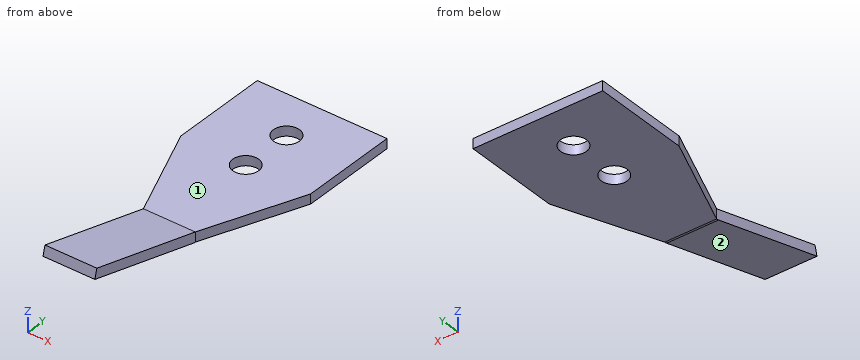
from build123d import *

# Parameters (mm, degrees)
SKETCH1_W           = 200
SKETCH1_H           = 300
SKETCH1_R           = 20
BOSS_EXTRUDE1_DEPTH = 15
CUT_EXTRUDE1_DEPTH  = 15
SKETCH3_W           = 80
SKETCH3_H           = 15
REVOLVE1_ANGLE      = 15
SKETCH4_W           = 80
SKETCH4_H           = 15
BOSS_EXTRUDE3_DEPTH = 200


with BuildPart() as part:
    # Sketch1 → Boss-Extrude1 (new body)
    with BuildSketch(Plane.XY):
        with Locations((-100, 150)):
            Rectangle(SKETCH1_W, SKETCH1_H)
        with Locations((-100, 230)):
            Circle(SKETCH1_R, mode=Mode.SUBTRACT)
        with Locations((-100, 150)):
            Circle(SKETCH1_R, mode=Mode.SUBTRACT)
    extrude(amount=BOSS_EXTRUDE1_DEPTH)

    # Sketch2 → Cut-Extrude1 (cut)
    with BuildSketch(Plane(origin=(0, 0, 0), x_dir=(-1, 0, 0), z_dir=(0, 0, -1))):
        Polygon((0, 0), (60, 0), (0, 150), align=None)
        Polygon((200, 0), (140, 0), (200, 150), align=None)
    extrude(amount=-CUT_EXTRUDE1_DEPTH, mode=Mode.SUBTRACT)

    # Sketch3 → Revolve1 (revolve)
    with BuildSketch(Plane.XZ):
        with Locations((-100, 7.5)):
            Rectangle(SKETCH3_W, SKETCH3_H)
    revolve(axis=Axis((-60, 0, 15), (-1, 0, 0)), revolution_arc=REVOLVE1_ANGLE)

    # Sketch4 → Boss-Extrude3 (add)
    with BuildSketch(Plane(origin=(0, -3.75, 1.004809472), x_dir=(1, 0, 0), z_dir=(0, -0.9659258262890681, 0.25881904510252135))):
        with Locations((-100, 6.988887394)):
            Rectangle(SKETCH4_W, SKETCH4_H)
    extrude(amount=BOSS_EXTRUDE3_DEPTH)


solid = part.part
Verification items for the finished model (mm, model axes). Face numbers are marked on the shaded views. A direction names the side the tool comes from. Give positions to 0.01 mm unless a question says otherwise; leave off trailing zeros. Order: outer loops, then holes, each group sorted by start corner. A loop starts at its lowest first (then second) coordinate and runs counter-clockwise, first axis right, second up. Notation, with made-up numbers: M 84.25,46.25 L 106.25,46.25 A15 ccw 106.25,64.25 Z; hole C -15.75,-21.5 d5. An arc over 180 degrees is marked long. Answer as a JSON object with one key per item and string values. Group by question number.
1) Cross-section at A-A (y = 230). Enter the section's corners in (x, z), then the cut area to 3 significant figures.
2) Cross-section at D-D (x = -67.5). Enter the section's corners in (y, z).
3) Cross-section at B-B (x = -100). Enter the section's corners in (y, z).
4) Access from +Z, -Z, +X, -X, +Y, -Y to the whole of each face (thin tool, end or side, straight path). Record for the marked faces 1 and 2.
5) Scan lines: line 1 along Z through (x, y) = (-13.5, 225); line 2 along X through (y, z) = (247, 5); line 3 along Z through (x, y) = (-108, -82.5). Record each from-to range of solid material in increasing order. Write a range as [from, to].
6) Depth check by flat-ended pin: pin 1 Ø20 at (y, z) = (-54, 27.5) entering from +X; pin 2 Ø8 at (x, y) = (-69.5, 69) entering from +Z. Enter the tip coordinate at first touch or a pass-through.
7) Cross-section at C-C (z = 10). Enter the section's corners in (x, y), then the cut area to 3 significant figures.
Result sheet:
{
 "1": {"outline": "M -200,0 L -120,0 L -120,15 L -200,15 Z; M -80,0 L 0,0 L 0,15 L -80,15 Z", "area": "2,400 mm2"},
 "2": {"outline": "M -197.07,52.27 L -3.88,0.51 A15 ccw 0,0 L 300,0 L 300,15 L 0,15 L -193.19,66.76 Z"},
 "3": {"outline": "M -197.07,52.27 L -3.88,0.51 A15 ccw 0,0 L 130,0 L 130,15 L 0,15 L -193.19,66.76 Z; M 170,0 L 210,0 L 210,15 L 170,15 Z; M 250,0 L 300,0 L 300,15 L 250,15 Z"},
 "4": {"face 1": "+Z, +X, -X, +Y", "face 2": "-Z, +X, -X, -Y"},
 "5": {"line 1": "z = [0, 15]", "line 2": "x = [-200, -110.54], [-89.46, 0]", "line 3": "z = [21.58, 37.11]"},
 "6": {"pin 1": "stops at x = -60", "pin 2": "stops at z = 15"},
 "7": {"outline": "M -200,150 L -140,0 L -140,-39.3 L -60,-39.3 L -60,0 L 0,150 L 0,300 L -200,300 Z; hole C -100,150 d40; hole C -100,230 d40", "area": "51,600 mm2"}
}
